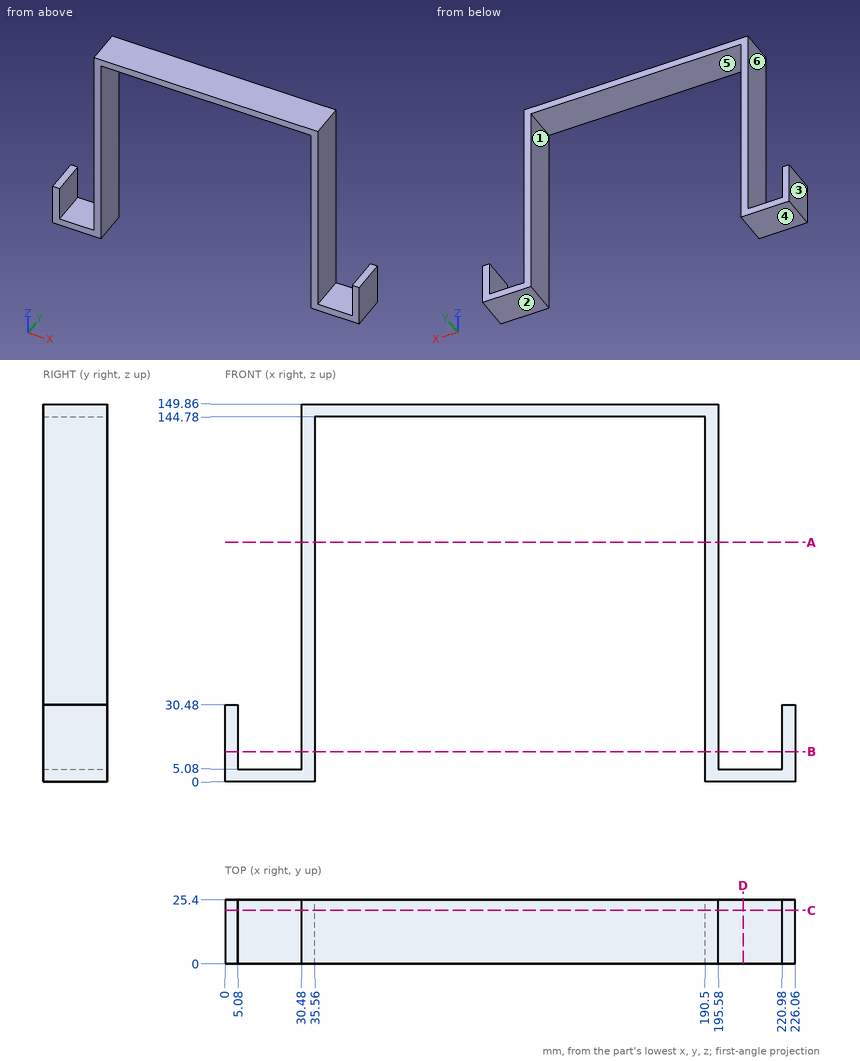
Can you work these out from the drawing? Everything is in mm from the part's minimum corner. A direction names the side the tool comes from. Round coordinates to 2 decimals unless told otherwise and drop trailing zeros. Loops run counter-clockwise (first coordinate to the right, second up) from the corner with the lowest first, then second, coordinate; pieces in that order, holes last. Notation, with made-up numbers: (64.25, 87.5) - (85.25, 87.5) arc R17 cw to (85.25, 110.5) - close; hole circle Ø7 at (59, 0). An arc over 180 degrees is marked (long way). Write item = value, one per line. Start each with the question number.
(1) If we section it at A-A (z = 95): Please give me the cut outline in (x, y), and give its area (3 significant figures).
(2) If we section it at C-C (y = 21.25): Please give me the cut outline in (x, z), and give its area (3 significant figures).
(3) For the marked faces 4, 5 and 6, which set-ups out of +Z, -Z, +X, -X, +Y, -Y let a thin tool reach every point of the face, with its end or its side?
(4) If I drill on probe 1 along X at (y, z) = (14, 25.5); probe 2 along X at (y, z) = (18.5, 100); probe 3 along Z at (x, y) = (139, 17.5), over which ranges is the centre line in solid material (lowest first)? Write a range as [from, to].
(5) If we mould it in two halves opening along X, with no side actions, what happens to the marked faces 1, 2 and 3? For each: released by +X, released by -X, zero draft, split by the parting line, or undercut.
(6) For P1, Ø2, axis at y = 21, z = 92, coming from the -X side; P2, Ø12.5, axis at y = 18, z = 85, coming from the +X side; P3, Ø4, axis at x = 223.5, y = 11.5, coming from the +Z side, each with a flat end and sliding along its axis, tell me the tip position at first contact or that it passes through.
(7) If we section it at D-D (x = 205.5): Please give me the cut outline in (y, z), and give its area (3 significant figures).
(8) If we section it at B-B (z = 12): Please give me the cut outline in (x, y), and give its area (3 significant figures).
Ans:
q1.outline = (30.48, 0) - (35.56, 0) - (35.56, 25.4) - (30.48, 25.4) - close; (190.5, 0) - (195.58, 0) - (195.58, 25.4) - (190.5, 25.4) - close
q1.area = 258 mm²
q2.outline = (0, 0) - (35.56, 0) - (35.56, 144.78) - (190.5, 144.78) - (190.5, 0) - (226.06, 0) - (226.06, 30.48) - (220.98, 30.48) - (220.98, 5.08) - (195.58, 5.08) - (195.58, 149.86) - (30.48, 149.86) - (30.48, 5.08) - (5.08, 5.08) - (5.08, 30.48) - (0, 30.48) - close
q2.area = 2,880 mm²
q3.face_4 = -Z, +X, -X, +Y, -Y
q3.face_5 = -Z, +Y, -Y
q3.face_6 = +Z, +Y, -Y
q4.probe_1 = [0, 5.08], [30.48, 35.56], [190.5, 195.58], [220.98, 226.06]
q4.probe_2 = [30.48, 35.56], [190.5, 195.58]
q4.probe_3 = [144.78, 149.86]
q5.face_1 = undercut
q5.face_2 = zero draft
q5.face_3 = released by -X
q6.P1 = 30.48
q6.P2 = 195.58
q6.P3 = 30.48
q7.outline = (0, 0) - (25.4, 0) - (25.4, 5.08) - (0, 5.08) - close
q7.area = 129 mm²
q8.outline = (0, 0) - (5.08, 0) - (5.08, 25.4) - (0, 25.4) - close; (30.48, 0) - (35.56, 0) - (35.56, 25.4) - (30.48, 25.4) - close; (190.5, 0) - (195.58, 0) - (195.58, 25.4) - (190.5, 25.4) - close; (220.98, 0) - (226.06, 0) - (226.06, 25.4) - (220.98, 25.4) - close
q8.area = 516 mm²
